The listing builds one solid part. Answer for the finished solid, in the listing's coordinates (mm). Round coordinates to 2 decimals unless told otherwise and drop trailing zeros. Write each loop counter-clockwise with the first axis right and the second up, starting at its lowest first coordinate (ties: lowest second). Pieces come first, ordered by that corner, then holes. Notation, with made-up numbers: M 11,84.25 L 39,84.25 A21 ccw 39,104.25 Z; hole C 86.25,31.25 d9. An arc over 180 degrees is marked long. Put each result on its own line as item: value. Start each with the question number.
```python
from build123d import *

# Parameters (mm, degrees)
BOSS_EXTRUDE1_DEPTH = 2
CUT_EXTRUDE2_DEPTH  = 2
CIRPATTERN1_COUNT   = 7
CIRPATTERN1_ANGLE   = 180
CUT_EXTRUDE3_DEPTH  = 2
CIRPATTERN2_COUNT   = 6
CIRPATTERN2_ANGLE   = 150
SKETCH5_R           = 2.5
CUT_EXTRUDE4_DEPTH  = 2
SKETCH6_R           = 1.15
CUT_EXTRUDE5_DEPTH  = 2


with BuildPart() as part:
    # Sketch1 → Boss-Extrude1 (new body)
    # profile 1 of 2: a face of its own
    with BuildSketch(Plane.XY):
        with BuildLine():
            ThreePointArc((40, 0), (0, -40), (-40, 0))
            Line((-40, 0), (-40, 15))
            Line((-40, 15), (40, 15))
            Line((40, 15), (40, 0))
        make_face()
        with BuildLine():
            ThreePointArc((-27.5, -1.25), (-26.25, 0), (-27.5, 1.25))
            Line((-27.5, 1.25), (-33.065653226, 1.25))
            Line((-33.065653226, 1.25), (-36.5, 0))
            Line((-36.5, 0), (-33.065653226, -1.25))
            Line((-33.065653226, -1.25), (-27.5, -1.25))
        make_face(mode=Mode.SUBTRACT)
    # profile 2 of 2: a face of its own
    with BuildSketch(Plane.XY):
        with BuildLine():
            Line((-33.065653226, -1.25), (-27.5, -1.25))
            ThreePointArc((-27.5, -1.25), (-26.25, 0), (-27.5, 1.25))
            Line((-27.5, 1.25), (-33.065653226, 1.25))
            Line((-33.065653226, 1.25), (-36.5, 0))
            Line((-36.5, 0), (-33.065653226, -1.25))
        make_face()
    extrude(amount=BOSS_EXTRUDE1_DEPTH)

    # Sketch2 → Cut-Extrude2 (cut)
    with BuildSketch(Plane.XY.offset(2)):
        with BuildLine():
            Line((-33.065653226, -1.25), (-27.5, -1.25))
            ThreePointArc((-27.5, -1.25), (-26.25, 0), (-27.5, 1.25))
            Line((-27.5, 1.25), (-33.065653226, 1.25))
            Line((-33.065653226, 1.25), (-36.5, 0))
            Line((-36.5, 0), (-33.065653226, -1.25))
        make_face()
    cut_extrude2 = extrude(amount=-CUT_EXTRUDE2_DEPTH, mode=Mode.SUBTRACT)

    # CirPattern1: Cut-Extrude2 ×7 about axis
    cirpattern1_axis = Axis((0, 0, 0), (0, 0, 1))
    for i in range(1, CIRPATTERN1_COUNT):
        add(cut_extrude2.rotate(cirpattern1_axis, i * CIRPATTERN1_ANGLE / (CIRPATTERN1_COUNT - 1)), mode=Mode.SUBTRACT)

    # Sketch4 → Cut-Extrude3 (cut)
    with BuildSketch(Plane.XY.offset(2)):
        with BuildLine():
            Line((-26.355904987, -7.890264401), (-31.185534118, -9.184359627))
            ThreePointArc((-31.185534118, -9.184359627), (-32.165330015, -8.618674202), (-31.59964459, -7.638878305))
            Line((-31.59964459, -7.638878305), (-26.770015459, -6.344783079))
            ThreePointArc((-26.770015459, -6.344783079), (-25.790219562, -6.910468504), (-26.355904987, -7.890264401))
        make_face()
    cut_extrude3 = extrude(amount=-CUT_EXTRUDE3_DEPTH, mode=Mode.SUBTRACT)

    # CirPattern2: Cut-Extrude3 ×6 about axis
    cirpattern2_axis = Axis((0, 0, 0), (0, 0, 1))
    for i in range(1, CIRPATTERN2_COUNT):
        add(cut_extrude3.rotate(cirpattern2_axis, i * CIRPATTERN2_ANGLE / (CIRPATTERN2_COUNT - 1)), mode=Mode.SUBTRACT)

    # Sketch5 → Cut-Extrude4 (cut)
    with BuildSketch(Plane.XY.offset(2)):
        Circle(SKETCH5_R)
    extrude(amount=-CUT_EXTRUDE4_DEPTH, mode=Mode.SUBTRACT)

    # Sketch6 → Cut-Extrude5 (cut)
    with BuildSketch(Plane.XY.offset(2)):
        with Locations((-20, 10)):
            Circle(SKETCH6_R)
        with Locations((20, 10)):
            Circle(SKETCH6_R)
    extrude(amount=-CUT_EXTRUDE5_DEPTH, mode=Mode.SUBTRACT)


solid = part.part
```
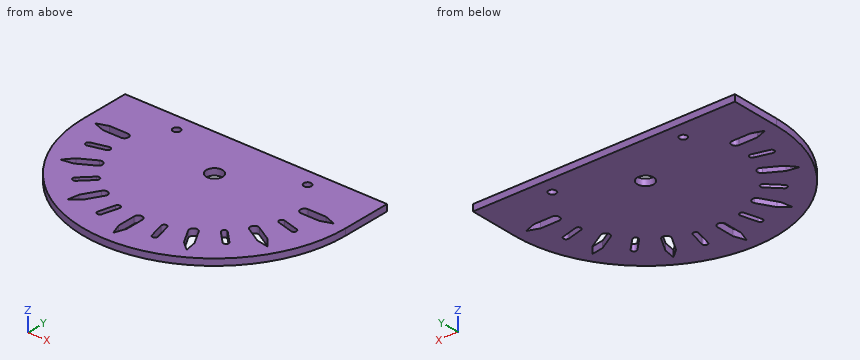
Item 1: Section C-C (z = 1.3) is taken. Count the separate pieces of the cut face and the enclosed holes in it, and give its area (3 significant figures).
Item 2: Flat-ended cylindrical pins translate along their axes: pin 1 (1 mm diameter, centred on x = 31.5, z = 1.5, fed in from -Y); pin 2 (0.6 mm diameter, centred on y = -31.5, z = 1, fed in from -X). Find the tip coordinate at first contact, or state that the pin passes through.
Item 3: Section B-B (x = -13.75) is taken. Give the vertices of the cut face in (y, z), and give its area (3 significant figures).
Item 4: Consider line 1 along X through (y, z) = (-32, 0.45); line 2 along Y through (x, z) = (26, 0.2); line 3 along Y through (x, z) = (34, 0.4). Determine where each line is inside the solid, lowest interval first. Write a range as [from, to].
Item 5: Section A-A (y = 10) is taken. Give the vertices of the cut face in (x, z).
Output values:
1. separate pieces: 1
1. enclosed holes: 16
1. area: 3,480 mm^2
2. pin 1: stops at y = -25.28
2. pin 2: stops at x = -25.03
3. outline: M -37.56,0 L -26.32,0 L -26.32,2 L -37.56,2 Z; M -22.57,0 L 15,0 L 15,2 L -22.57,2 Z
3. area: 97.6 mm^2
4. line 1: x = [-24, -8.93], [-7.89, -1.25], [1.25, 7.89], [8.93, 24]
4. line 2: y = [-30.4, -16.45], [-13.57, -7.69], [-6.55, 15]
4. line 3: y = [-21.07, -0.91], [0.91, 15]
5. outline: M -40,0 L -21.15,0 L -21.15,2 L -40,2 Z; M -18.85,0 L 18.85,0 L 18.85,2 L -18.85,2 Z; M 21.15,0 L 40,0 L 40,2 L 21.15,2 Z
